```python
from build123d import *

# Parameters (mm, degrees)
SKETCH1_W               = 272
SKETCH1_H               = 5
BOSS_EXTRUDE1_DEPTH     = 28
SKETCH2_W               = 8
SKETCH2_H               = 28
BOSS_EXTRUDE2_DEPTH     = 15
CUT_EXTRUDE1_DEPTH      = 274.996806551
CUT_EXTRUDE1_DEPTH_BACK = 274.996806551
SKETCH3_W               = 15
SKETCH3_H               = 12
FILLET1_R               = 1
CUT_EXTRUDE2_DEPTH      = 274.996806551
CUT_EXTRUDE2_DEPTH_BACK = 274.996806551
SKETCH4_R               = 2


with BuildPart() as part:
    # Sketch1 → Boss-Extrude1 (new body)
    with BuildSketch(Plane(origin=(0, 0, 0), x_dir=(1, 0, 0), z_dir=(0, 1, 0))):
        Rectangle(SKETCH1_W, SKETCH1_H)
    extrude(amount=BOSS_EXTRUDE1_DEPTH)

    # Sketch2 → Boss-Extrude2 (add)
    with BuildSketch(Plane(origin=(0, 0, -2.5), x_dir=(-1, 0, 0), z_dir=(0, 0, -1))):
        with Locations((-132, 14)):
            Rectangle(SKETCH2_W, SKETCH2_H)
        with Locations((132, 14)):
            Rectangle(SKETCH2_W, SKETCH2_H)
    extrude(amount=BOSS_EXTRUDE2_DEPTH)

    # Sketch3 → Cut-Extrude1 (cut, two sides: drawn at the far end of the back side and taken through both)
    with BuildSketch(Plane(origin=(136, 0, 0), x_dir=(0, 0, -1), z_dir=(1, 0, 0)).offset(-CUT_EXTRUDE1_DEPTH_BACK)):
        with Locations((10, 14)):
            Rectangle(SKETCH3_W, SKETCH3_H)
    extrude(amount=CUT_EXTRUDE1_DEPTH + CUT_EXTRUDE1_DEPTH_BACK, mode=Mode.SUBTRACT)

    # Fillet1
    fillet1_edges = [part.edges().sort_by_distance(p)[0] for p in [
        (0, 0, -2.5),
        (0, 28, -2.5),
        (128, 4, -2.5),
        (128, 0, -10),
        (128, 28, -10),
        (128, 4, -17.5),
        (-128, 24, -2.5),
        (-128, 28, -10),
        (-128, 0, -10),
        (-128, 24, -17.5),
        (-128, 4, -17.5),
        (-128, 4, -2.5),
        (128, 24, -17.5),
        (128, 24, -2.5),
        (132, 8, -2.5),
        (-132, 8, -2.5),
        (132, 20, -2.5),
        (-132, 20, -2.5),
        (128, 8, -10),
        (-128, 8, -10),
        (128, 20, -10),
        (-128, 20, -10),
    ]]
    fillet(fillet1_edges, radius=FILLET1_R)

    # Sketch4 → Cut-Extrude2 (cut, two sides: drawn at the far end of the back side and taken through both)
    with BuildSketch(Plane(origin=(136, 0, 0), x_dir=(0, 0, -1), z_dir=(1, 0, 0)).offset(-CUT_EXTRUDE2_DEPTH_BACK)):
        with Locations((11.5, 24)):
            Circle(SKETCH4_R)
        with Locations((11.5, 4)):
            Circle(SKETCH4_R)
    extrude(amount=CUT_EXTRUDE2_DEPTH + CUT_EXTRUDE2_DEPTH_BACK, mode=Mode.SUBTRACT)


solid = part.part
```
Could you check a few things on this model? Use its own coordinates, in mm. A direction names the side the tool comes from. Give positions to 0.01 mm unless a question says otherwise; leave off trailing zeros. Order: outer loops, then holes, each group sorted by start corner. A loop starts at its lowest first (then second) coordinate and runs counter-clockwise, first axis right, second up.
Q1. If I drill on line 1 along Y through (x, z) = (133.75, -11.5); line 2 along X through (y, z) = (2.5, -9.25); line 3 along Z through (x, y) = (-132, 4), over which ranges is the centre line in solid material (lowest first)?
Q2. Suppose I cut it at C-C, the plane x = 56. Write out the boundary of the cut face in (y, z), and give its area (3 significant figures).
Q3. For faces 4 (the flat face through (-132, 4, -17.5)), 5 (the flat face through (-133, 20, -10)), 6 (the flat face through (-128, 4, -8)), which set-ups out of +Z, -Z, +X, -X, +Y, -Y let a thin tool reach every point of the face, with its end or its side?
Q4. Suppose I cut it at B-B, the plane y = 15.75. Write out the boundary of the cut face in (x, z).
Q5. I'm going to push a flat-ended pin straight in: P1, Ø2, axis at x = 14, y = 21.5, coming from the -Z side. Where does the tip first touch, or does it pass through?
Q6. Suppose I cut it at A-A, the plane z = -6.5. Write out the boundary of the cut face in (x, y), and give its area (3 significant figures).
Q7. We'd pull the mould along X, two halves only. Please class faces 1 (the flat face through (133, 24, -17.5)), 2 (the flat face through (136, 14, -1)), 3 (the flat face through (-2, 14, -2.5)): +X half, -X half, draft (parallel to the pull), parting line (faces both ways), or undercut.
Solution:
1. line 1: y = 0 to 2, 6 to 8, 20 to 22, 26 to 28
1. line 2: x = -136 to -128, 128 to 136
1. line 3: z = -17.5 to -13.5, -9.5 to 2.5
2. outline: (0, -1.5) arc R1 ccw to (1, -2.5) - (27, -2.5) arc R1 ccw to (28, -1.5) - (28, 2.5) - (0, 2.5) - close
2. area: 140 mm2
3. face 4: -Z, +X, -X, +Y, -Y
3. face 5: -Z, +X, -X
3. face 6: -Z, +Y, -Y
4. outline: (-136, -2.5) - (136, -2.5) - (136, 2.5) - (-136, 2.5) - close
5. P1: stops at z = -2.5
6. outline: (-136, 0) - (-129, 0) arc R1 ccw to (-128, 1) - (-128, 7) arc R1 ccw to (-129, 8) - (-136, 8) - close; (-136, 20) - (-129, 20) arc R1 ccw to (-128, 21) - (-128, 27) arc R1 ccw to (-129, 28) - (-136, 28) - close; (128, 1) arc R1 ccw to (129, 0) - (136, 0) - (136, 8) - (129, 8) arc R1 ccw to (128, 7) - close; (128, 21) arc R1 ccw to (129, 20) - (136, 20) - (136, 28) - (129, 28) arc R1 ccw to (128, 27) - close
6. area: 254 mm2
7. face 1: draft
7. face 2: +X half
7. face 3: undercut
